The listing builds one solid part. Answer for the finished solid, in the listing's coordinates (mm). A direction names the side the tool comes from. Coordinates: 2 decimals unless noted, no trailing zeros. Write each loop counter-clockwise with the first axis right and the second up, starting at its lowest first coordinate (ties: lowest second). Pieces come first, ordered by that corner, then holes.
(1) For a pull along X with two mould halves and no side action, classify faces 5 (the flat face through (28.296, 2, -24)), 6 (the cylindrical face through (45.3, -16.56, 15.18)), 7 (the flat face through (26.721, 12, -6)), 8 (the cylindrical face through (37.09, 21.51, 0.08)) as +X half, -X half, draft (parallel to the pull), parting line (faces both ways), or undercut.
(2) Given P1, Ø8, axis at x = 21, y = 12.5, coming from the +Z side; P2, Ø2, axis at x = 8, y = -4.5, coming from the +Z side; P3, Ø4.5, axis at y = -19.74, z = 0, coming from the -X side, each flat-ended and moving along its own axis, determine where each tip first touches the part or whether it passes through.
(3) The part is cut by section C-C on x = 22.5. Determine the outline of the cut face in (y, z).
(4) Straight lines are drawn through the part: line 1 (Z direction, x = 33, y = 0); line 2 (Z direction, x = 32, y = -1); line 3 (X direction, y = 7.5, z = -23). For each, find the intervals that lie inside material, in ascending order.
(5) Which of the six approach directions +Z, -Z, +X, -X, +Y, -Y give full straight-line access (tool end or side, diameter ignored) to faces 1 (the cylindrical face through (37.09, 0.23, 21.5)), 2 (the cylindrical face through (13.56, -2.75, -12.4)), 3 (the cylindrical face through (36.26, -18.897, -14.49)), 4 (the flat face through (44.45, -14, -18))?
(6) The part is cut by section A-A on y = 0. Give the number of separate pieces and of enclosed holes in the cut face, plus the area to 3 significant figures.
from build123d import *

# Parameters (mm, degrees)
F0_R      = 12.7
F1_DEPTH  = 26.7208
F2_R      = 26.924
F2_R_2    = 12.7
F3_DEPTH  = 1.5748
F4_R      = 23.8125
F5_DEPTH  = 16.1544
F6_R      = 22.4663
F7_DEPTH  = 1.7272
F8_R      = 23.8125
F9_DEPTH  = 1.5748
F10_SIZE  = 0.762
F11_SIZE  = 0.762
F12_R     = 1.778
F13_DEPTH = 21.0322


with BuildPart() as f1:
    # F0 (on Right) → F1 (new body)
    with BuildSketch(Plane.YZ):
        Circle(F0_R)
    extrude(amount=F1_DEPTH)

    # F2 (on face) → F3 (join)
    with BuildSketch(Plane.YZ.offset(26.7208)):
        Circle(F2_R)
        Circle(F2_R_2, mode=Mode.SUBTRACT)
        Circle(F2_R_2)
    extrude(amount=F3_DEPTH)

    # F4 (on face) → F5 (join)
    with BuildSketch(Plane.YZ.offset(28.2956)):
        Circle(F4_R)
    extrude(amount=F5_DEPTH)

    # F6 (on face) → F7 (join)
    with BuildSketch(Plane.YZ.offset(44.45)):
        Circle(F6_R)
    extrude(amount=F7_DEPTH)

    # F8 (on face) → F9 (join)
    with BuildSketch(Plane.YZ.offset(46.1772)):
        Circle(F8_R)
    extrude(amount=F9_DEPTH)

    # F10
    f10_edges = [f1.edges().sort_by_distance(p)[0] for p in [
        (47.752, -23.8125, 0),
    ]]
    chamfer(f10_edges, length=F10_SIZE)

    # F11
    f11_edges = [f1.edges().sort_by_distance(p)[0] for p in [
        (0, -12.7, 0),
    ]]
    chamfer(f11_edges, length=F11_SIZE)

    # F12 (on face) → F13 (cut, through all)
    with BuildSketch(Plane(origin=(26.7208, 0, 0), x_dir=(0, -1, 0), z_dir=(-1, 0, 0))):
        with Locations((0, 19.7358)):
            Circle(F12_R)
        with Locations((19.7358, 0)):
            Circle(F12_R)
        with Locations((0, -19.7358)):
            Circle(F12_R)
        with Locations((-19.7358, 0)):
            Circle(F12_R)
    extrude(amount=-F13_DEPTH, mode=Mode.SUBTRACT)


solid = f1.part
Model answer:
1. face 5: +X half
1. face 6: undercut
1. face 7: -X half
1. face 8: draft
2. P1: stops at z = 9.44
2. P2: stops at z = 12.21
2. P3: stops at x = 26.72
3. outline: circle Ø25.4 at (0, 0)
4. line 1: z = -23.81 to -21.51, -17.96 to 17.96, 21.51 to 23.81
4. line 2: z = -23.79 to -21.21, -18.27 to 18.27, 21.21 to 23.79
4. line 3: x = 26.72 to 28.3
5. face 1: +X, -X
5. face 2: -X
5. face 3: +X
5. face 4: none
6. separate pieces: 3
6. enclosed holes: 0
6. area: 1,530 mm2
